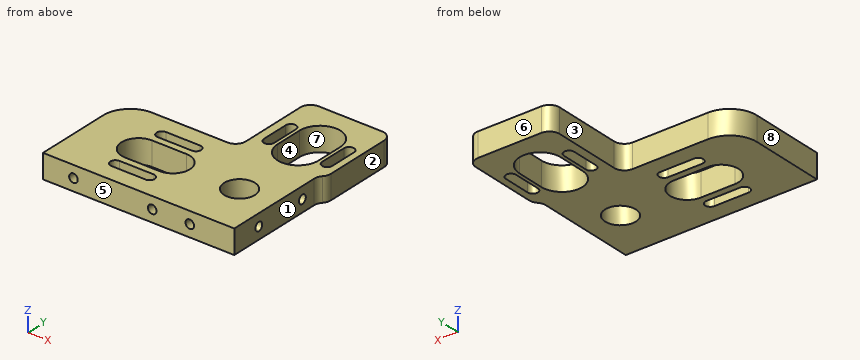
Autodesk Inventor part; units mm, degrees
ref_plane "YZ Plane" through (0, 0, 0) normal (1, 0, 0) x (0, 1, 0)
ref_plane "XZ Plane" through (0, 0, 0) normal (0, 1, 0) x (-1, 0, 0)
ref_plane "XY Plane" through (0, 0, 0) normal (0, 0, 1) x (1, 0, 0)
sketch "Esquisse1" plane through (0, 0, 0) normal (0, 0, 1) x (1, 0, 0)
  point P0 (0, 0)
sketch "Esquisse2" plane through (0, 0, 0) normal (0, 0, 1) x (1, 0, 0)
  line L0 (0, 56) -> (57.5, 56)
  line L1 (57.5, 56) -> (57.5, 0)
  line L2 (57.5, 0) -> (0, 0)
  line L3 (0, 0) -> (0, 56)
  dimension "d0" = 57.5
  dimension "d1" = 56
extrude "Extrusion1" add sketch "Esquisse2" along normal blind 7
sketch "Esquisse3" plane through (0, 0, 7) normal (0, 0, 1) x (1, 0, 0)
  line L0 (57.5, 56) -> (0, 56)
  line L1 (0, 56) -> (33, 56)
  line L2 (33, 56) -> (33, 30)
  line L3 (33, 30) -> (0, 30)
  line L4 (0, 30) -> (0, 56)
  line L5 (0, 0) -> (57.5, 0)
  line L6 (57.5, 0) -> (57.5, 56)
  dimension "d5" = 30
  dimension "d6" = 24.5
extrude "Extrusion2" cut sketch "Esquisse3" against normal through all
sketch "Esquisse4" plane through (0, 0, 7) normal (0, 0, 1) x (1, 0, 0)
  circle A0 centre (45.5, 15) radius 4.5
  line L0 (16, 15) -> (26, 15) construction
  line L1 (16, 10) -> (26, 10)
  line L2 (26, 20) -> (16, 20)
  arc A1 (16, 20) -> (16, 10) centre (16, 15) ccw
  arc A2 (26, 10) -> (26, 20) centre (26, 15) ccw
  line L3 (16, 23.5) -> (26, 23.5) construction
  line L4 (16, 22) -> (26, 22)
  line L5 (26, 25) -> (16, 25)
  arc A3 (16, 25) -> (16, 22) centre (16, 23.5) ccw
  arc A4 (26, 22) -> (26, 25) centre (26, 23.5) ccw
  line L6 (16, 6.5) -> (26, 6.5) construction
  line L7 (16, 5) -> (26, 5)
  line L8 (26, 8) -> (16, 8)
  arc A5 (16, 8) -> (16, 5) centre (16, 6.5) ccw
  arc A6 (26, 5) -> (26, 8) centre (26, 6.5) ccw
  line L9 (45.5, 44.5) -> (45.5, 36.5) construction
  line L10 (51.5, 44.5) -> (51.5, 36.5)
  line L11 (39.5, 36.5) -> (39.5, 44.5)
  arc A7 (51.5, 44.5) -> (39.5, 44.5) centre (45.5, 44.5) ccw
  arc A8 (39.5, 36.5) -> (51.5, 36.5) centre (45.5, 36.5) ccw
  line L12 (37, 44.5) -> (37, 36.5) construction
  line L13 (38.5, 44.5) -> (38.5, 36.5)
  line L14 (35.5, 36.5) -> (35.5, 44.5)
  arc A9 (38.5, 44.5) -> (35.5, 44.5) centre (37, 44.5) ccw
  arc A10 (35.5, 36.5) -> (38.5, 36.5) centre (37, 36.5) ccw
  line L15 (54, 44.5) -> (54, 36.5) construction
  line L16 (52.5, 44.5) -> (52.5, 36.5)
  line L17 (55.5, 36.5) -> (55.5, 44.5)
  arc A11 (55.5, 44.5) -> (52.5, 44.5) centre (54, 44.5) ccw
  arc A12 (52.5, 36.5) -> (55.5, 36.5) centre (54, 36.5) ccw
  line L18 (0, 0) -> (57.5, 0)
  line L19 (57.5, 0) -> (57.5, 56)
  line L20 (33, 56) -> (33, 30)
  line L21 (57.5, 56) -> (33, 56)
  line L22 (0, 30) -> (0, 0)
  point P0 (21, 15)
  point P1 (21, 23.5)
  point P2 (21, 6.5)
  point P3 (45.5, 40.5)
  point P4 (37, 40.5)
  point P5 (54, 40.5)
  dimension "d9" = 12
  dimension "d10" = 3
  dimension "d11" = 3
  dimension "d12" = 3
  dimension "d13" = 3
  dimension "d14" = 10
  dimension "d15" = 9
  dimension "d19" = 13
  dimension "d20" = 13
  dimension "d21" = 20
  dimension "d22" = 20
  dimension "d23" = 11
  dimension "d24" = 11
  dimension "d25" = 1
  dimension "d26" = 1
  dimension "d27" = 2
  dimension "d28" = 2
  dimension "d30" = 15
  dimension "d31" = 12
  dimension "d32" = 5
  dimension "d33" = 2.5
  dimension "d34" = 5.5
  dimension "d37" = 16
  dimension "d38" = 0
  dimension "d39" = 0
  dimension "d40" = 0
  dimension "d41" = 0
extrude "Extrusion3" cut sketch "Esquisse4" against normal through all
fillet "Congé1" radius 8 1 edges at (0, 30, 3.5)
fillet "Congé2" radius 3 3 edges at (33, 56, 3.5) (57.5, 56, 3.5) (33, 30, 3.5)
sketch "Esquisse5" plane through (0, 0, 7) normal (0, 0, 1) x (1, 0, 0)
  line L0 (57.5, 32) -> (55.9, 32)
  line L1 (55.9, 32) -> (55.9, 0)
  line L2 (55.9, 0) -> (57.5, 0)
  line L3 (57.5, 0) -> (57.5, 32)
  line L4 (57.5, 0) -> (57.5, 53)
  line L5 (0, 0) -> (57.5, 0)
  dimension "d46" = 1.6
  dimension "d47" = 32
extrude "Extrusion4" cut sketch "Esquisse5" against normal through all
fillet "Congé3" radius 3 2 edges at (55.9, 32, 3.5) (57.5, 32, 3.5)
sketch "Esquisse6" plane through (55.9, 0, 7) normal (1, 0, 0) x (0, 0, -1)
  circle A0 centre (3.5, 9) radius 1.25
  circle A1 centre (3.5, 25) radius 1.25
  line L0 (7, 29.3467) -> (7, 0)
  line L1 (7, 0) -> (0, 0)
  dimension "d51" = 2.5
  dimension "d52" = 2.5
  dimension "d53" = 3.5
  dimension "d54" = 3.5
  dimension "d55" = 16
  dimension "d56" = 9
extrude "Extrusion5" cut sketch "Esquisse6" against normal blind 5
sketch "Esquisse7" plane through (0, 0, 0) normal (0, -1, 0) x (1, 0, 0)
  circle A0 centre (8.9, 3.5) radius 1.25
  circle A1 centre (31.9, 3.5) radius 1.25
  circle A2 centre (42.9, 3.5) radius 1.25
  line L0 (55.9, 0) -> (0, 0)
  line L1 (57.5, 0) -> (57.5, 7)
  line L2 (0, 0) -> (0, 7)
  line L3 (55.9, 0) -> (55.9, 7)
  dimension "d59" = 2.5
  dimension "d60" = 2.5
  dimension "d61" = 2.5
  dimension "d62" = 3.5
  dimension "d63" = 3.5
  dimension "d64" = 3.5
  dimension "d65" = 11
  dimension "d70" = 13
  dimension "d71" = 23
extrude "Extrusion6" cut sketch "Esquisse7" against normal blind 5
equation "\"d52\" = d51"
equation "\"d54\" = d53"
equation "\"d60\" = d59"
equation "\"d61\" = d59"
equation "\"d63\" = d62"
equation "\"d64\" = d62"
properties part number "SupportMoteur" material "Plastique ABS"
Geometry: final body of the model. Coordinates: model frame, mm. Face numbers are marked on the shaded views. A direction names the side the tool comes from. Round coordinates to 2 decimals unless told otherwise and drop trailing zeros. Order: outer loops, then holes, each group sorted by start corner. A loop starts at its lowest first (then second) coordinate and runs counter-clockwise, first axis right, second up. Notation, with made-up numbers: (-5, 80) - (21, 80) arc R32 cw to (21, 112) - close; hole circle Ø8 at (6.5, 23). An arc over 180 degrees is marked (long way). Use CSV: the item, a comma, the result in double quotes. Start each with the question number.
Q1. Section query C-C (x = 37). Return loops of the section in (y, z).
Q2. Section query A-A (x = 45.5). Return loops of the section in (y, z).
Q3. First-contact query: pin 1 (3 mm diameter, centred on x = 8.9, z = 3.5, fed in from +Y); pin 2 (1 mm diameter, centred on y = 12, z = 3, fed in from +X); pin 3 (1.2 mm diameter, centred on y = 25, z = 3, fed in from +X). Flat tips, straight axial feed; report the tip coordinate or a pass-through.
Q4. Material intervals for line 1 along X through (y, z) = (40, 2); line 2 along Y through (x, z) = (45.5, 3); line 3 along Y through (x, z) = (21.5, 3.5), sorted ascending. Write a range as from..to.
Q5. Mould query, pull axis X, two halves, no side actions, for the marked faces 6, 7 and 8. Classes: +X half, -X half, draft (parallel to the pull), parting line (faces both ways), or undercut.
Q6. Section query D-D (y = 43.5). Return loops of the section in (x, z), and give its area (3 significant figures).
Q7. Access query for the marked faces 1, 2, 3, 4 and 5. Directions: +Z, -Z, +X, -X, +Y, -Y. A direction counts if a zero-diameter tool reaches every point of the face in a straight line with its end or side. Return the directions, or none.
Q8. Section query B-B (y = 6.5). Return loops of the section in (x, z).
Result set:
1,outline,"(0, 0) - (35, 0) - (35, 7) - (0, 7) - close; (46, 0) - (56, 0) - (56, 7) - (46, 7) - close"
2,outline,"(0, 0) - (10.5, 0) - (10.5, 7) - (0, 7) - close; (19.5, 0) - (30.5, 0) - (30.5, 7) - (19.5, 7) - close; (50.5, 0) - (56, 0) - (56, 7) - (50.5, 7) - close"
3,pin 1,"stops at y = 30"
3,pin 2,"stops at x = 55.9"
3,pin 3,"stops at x = 50.9"
4,line 1,"x = 33..35.5, 38.5..39.5, 51.5..52.5, 55.5..57.5"
4,line 2,"y = 0..10.5, 19.5..30.5, 50.5..56"
4,line 3,"y = 0..5, 8..10, 20..22, 25..30"
5,face 6,"draft"
5,face 7,"undercut"
5,face 8,"-X half"
6,outline,"(33, 0) - (35.5, 0) - (35.5, 7) - (33, 7) - close; (38.5, 0) - (39.5, 0) - (39.5, 7) - (38.5, 7) - close; (51.5, 0) - (52.5, 0) - (52.5, 7) - (51.5, 7) - close; (55.5, 0) - (57.5, 0) - (57.5, 7) - (55.5, 7) - close"
6,area,"45.5 mm2"
7,face 1,"+Z, -Z, +X, -Y"
7,face 2,"+Z, -Z, +X, +Y, -Y"
7,face 3,"+Z, -Z, -X, +Y"
7,face 4,"+Z, -Z"
7,face 5,"+Z, -Z, +X, -X, -Y"
8,outline,"(0, 0) - (14.5, 0) - (14.5, 7) - (0, 7) - close; (27.5, 0) - (55.9, 0) - (55.9, 7) - (27.5, 7) - close"
